Check sheet for the modelled part. Datum: model origin and axes. Units: mm. A direction names the side the tool comes from. Round coordinates to 2 decimals unless told otherwise and drop trailing zeros. Order: outer loops, then holes, each group sorted by start corner. A loop starts at its lowest first (then second) coordinate and runs counter-clockwise, first axis right, second up.
(1) Depth check by flat-ended pin: pin 1 (1.5 mm diameter, centred on x = 33.5, y = -4.5, fed in from +Z); pin 2 (2 mm diameter, centred on x = 8.5, z = 20.5, fed in from -Y); pin 3 (1.5 mm diameter, centred on x = -10.5, z = 6.5, fed in from -Y). Enter the tip coordinate at first touch or a pass-through.
(2) Sectioned sample at D-D, the plane z = -22. Enter the section's corners in (x, y).
(3) Thickness scan on probe 1 along Y at (x, z) = (14, -34); probe 2 along X at (y, z) = (-4.5, -33.5); probe 3 along Y at (x, z) = (-9, 46). Record the ranges inside material, lowest first.
(4) Sectioned sample at C-C, the plane x = -1.5. Enter the section's corners in (y, z).
(5) Sectioned sample at B-B, the plane z = 38. Enter the section's corners in (x, y), and give its area (3 significant figures).
(6) Sectioned sample at A-A, the plane z = -34. Enter the section's corners in (x, y), and give its area (3 significant figures).
(7) Mould release check, pull along Y, two halves, no side actions. Record for faces 5 (the flat face through (-17.785, -5, 40)), 6 (the flat face through (10, -10.414, 29)), 7 (the flat face through (-21.342, -5, 0)): released by +Y, released by -Y, zero draft, split by the parting line, or undercut.
(8) Tool access check on faces 1 (the flat face through (17, -10.414, -20)), 2 (the flat face through (9, 0, 1)), 3 (the flat face through (0, -5, -39)), 4 (the flat face through (-10, -7.194, 40)). Record the directions out of +Z, -Z, +X, -X, +Y, -Y that give a thin tool (end or side, any length) a straight path to the whole face; none if there is none.
```python
from build123d import *

# Parameters (mm, degrees)
F0_W        = 60.96
F0_H        = 104.14
F1_DEPTH    = 10.414
F2_W        = 60.96
F2_H        = 104.14
F2_R        = 17.78
F2_W_2      = 49.2147877812
F2_H_2      = 38.1
F3_DEPTH    = 0.508
F4_R        = 7.62
F5_DEPTH    = 0.254
F6_W        = 15.2469340246
F6_H        = 4.8402966931
F6_R        = 2.4201483466
F7_DEPTH    = 25.4
F8_T1_DEPTH = 35.306
F9_W        = 22.3395526409
F9_H        = 4.0701881517
F10_DEPTH   = 25.4


# Not quite as in the source:
# - a fillet or chamfer that OpenCascade refuses, or shapes differently, is made with other operations: its cross-section is extruded or revolved along the edge and cut away or added


with BuildPart() as f1:
    # F0 (on Front) → F1 (new body)
    with BuildSketch(Plane.XZ):
        with Locations((9.1376345801, 0.7195156068)):
            Rectangle(F0_W, F0_H)
    extrude(amount=F1_DEPTH)

    # F2 (on face) → F3 (cut)
    with BuildSketch(Plane.XZ.offset(10.414)):
        with Locations((9.1376345801, 0.7195156068)):
            Rectangle(F2_W, F2_H)
        with Locations((9.1376345801, -20.5781124532)):
            Circle(F2_R, mode=Mode.SUBTRACT)
        with Locations((10.3610083461, 28.4036870554)):
            Rectangle(F2_W_2, F2_H_2, mode=Mode.SUBTRACT)
    extrude(amount=-F3_DEPTH, mode=Mode.SUBTRACT)

    # F4 (on face) → F5 (join)
    with BuildSketch(Plane.XZ.offset(10.414)):
        with Locations((9.1376345801, -20.5781124532)):
            Circle(F4_R)
    extrude(amount=F5_DEPTH)

    # F6 (on face) → F7 (cut)
    with BuildSketch(Plane.XY.offset(52.7895156068)):
        with Locations((-10.1616705069, -4.773916211)):
            Rectangle(F6_W, F6_H)
        with Locations((33.7640233338, -4.773916211)):
            Circle(F6_R)
    extrude(amount=-F7_DEPTH, mode=Mode.SUBTRACT)

    # F8: fillet of radius 5.08 on 4 edges, made by hand

    # F8_s2 → F8_t1 (cut)
    with BuildSketch(Plane.XZ.offset(-12.7)):
        with BuildLine():
            ThreePointArc((39.6176345801, -46.2704843932), (38.1297370286, -49.8625868417), (34.5376345801, -51.3504843932))
            Line((34.5376345801, -51.3504843932), (39.6176345801, -51.3504843932))
            Line((39.6176345801, -51.3504843932), (39.6176345801, -46.2704843932))
        make_face()
        with BuildLine():
            ThreePointArc((-21.3423654199, -46.2704843932), (-19.8544678683, -49.8625868417), (-16.2623654199, -51.3504843932))
            Line((-16.2623654199, -51.3504843932), (-21.3423654199, -51.3504843932))
            Line((-21.3423654199, -51.3504843932), (-21.3423654199, -46.2704843932))
        make_face()
        with BuildLine():
            ThreePointArc((-16.2623654199, 52.7895156068), (-19.8544678683, 51.3016180552), (-21.3423654199, 47.7095156068))
            Line((-21.3423654199, 47.7095156068), (-21.3423654199, 52.7895156068))
            Line((-21.3423654199, 52.7895156068), (-16.2623654199, 52.7895156068))
        make_face()
        with BuildLine():
            ThreePointArc((34.5376345801, 52.7895156068), (38.1297370286, 51.3016180552), (39.6176345801, 47.7095156068))
            Line((39.6176345801, 47.7095156068), (39.6176345801, 52.7895156068))
            Line((39.6176345801, 52.7895156068), (34.5376345801, 52.7895156068))
        make_face()
    extrude(amount=F8_T1_DEPTH, mode=Mode.SUBTRACT)

    # F9 (on face) → F10 (cut)
    with BuildSketch(Plane(origin=(0, 0, -51.3504843932), x_dir=(1, 0, 0), z_dir=(0, 0, -1))):
        with Locations((11.1697763205, 4.9349990441)):
            Rectangle(F9_W, F9_H)
    extrude(amount=-F10_DEPTH, mode=Mode.SUBTRACT)


solid = f1.part
```
Derived:
1. pin 1: stops at z = 27.39
1. pin 2: stops at y = -10.41
1. pin 3: stops at y = -9.91
2. outline: (-21.34, -9.91) - (-8.59, -9.91) - (-8.59, -10.41) - (1.65, -10.41) - (1.65, -10.67) - (16.62, -10.67) - (16.62, -10.41) - (26.86, -10.41) - (26.86, -9.91) - (39.62, -9.91) - (39.62, 0) - (-21.34, 0) - close
3. probe 1: y = -10.41 to -6.97, -2.9 to 0
3. probe 2: x = -21.34 to 0, 22.34 to 39.62
3. probe 3: y = -10.41 to -7.19, -2.35 to 0
4. outline: (-10.41, -34.82) - (-9.91, -34.82) - (-9.91, -51.35) - (0, -51.35) - (0, 52.79) - (-9.91, 52.79) - (-9.91, 47.45) - (-10.41, 47.45) - (-10.41, 9.35) - (-9.91, 9.35) - (-9.91, -6.33) - (-10.41, -6.33) - close
5. outline: (-21.34, -9.91) - (-14.25, -9.91) - (-14.25, -10.41) - (34.97, -10.41) - (34.97, -9.91) - (39.62, -9.91) - (39.62, 0) - (-21.34, 0) - close; hole (-17.79, -7.19) - (-2.54, -7.19) - (-2.54, -2.35) - (-17.79, -2.35) - close; hole circle Ø4.84 at (33.76, -4.77)
5. area: 537 mm2
6. outline: (-21.34, -9.91) - (-2.52, -9.91) - (-2.52, -10.41) - (20.8, -10.41) - (20.8, -9.91) - (39.62, -9.91) - (39.62, 0) - (-21.34, 0) - close; hole (0, -6.97) - (22.34, -6.97) - (22.34, -2.9) - (0, -2.9) - close
6. area: 525 mm2
7. face 5: undercut
7. face 6: released by -Y
7. face 7: zero draft
8. face 1: -Y
8. face 2: +Z, -Z, +X, -X, +Y
8. face 3: -Z
8. face 4: +Z
